Geometry check sheet. Reference: the model listing, model coordinates, mm. A direction names the side the tool comes from. Round coordinates to 2 decimals unless told otherwise and drop trailing zeros. Order: outer loops, then holes, each group sorted by start corner. A loop starts at its lowest first (then second) coordinate and runs counter-clockwise, first axis right, second up. Notation, with made-up numbers: (10, 7.5) - (66, 7.5) arc R27 ccw to (66, 25.5) - close; hole circle Ø7 at (32.5, 49.5). An arc over 180 degrees is marked (long way). Write each question's results on one line, items separated by ' | '.
```python
from build123d import *

# Parameters (mm, degrees)
ESBO_O1_R                = 6.25
RESSALTO_EXTRUS_O1_DEPTH = 16.9
ESBO_O2_R                = 12
RESSALTO_EXTRUS_O2_DEPTH = 1.3
ESBO_O3_R                = 1.6
CORTE_EXTRUS_O1_DEPTH    = 25.884533349
ESBO_O4_R                = 2.45
RESSALTO_EXTRUS_O3_DEPTH = 4.1
ESBO_O5_R                = 0.6
CORTE_EXTRUS_O2_DEPTH    = 1
ESBO_O7_R                = 0.6
CORTE_EXTRUS_O3_DEPTH    = 1


with BuildPart() as part:
    # Esboço1 → Ressalto-extrusão1 (new body)
    with BuildSketch(Plane(origin=(0, 0, 0), x_dir=(1, 0, 0), z_dir=(0, 1, 0))):
        with Locations(Location((0, 0, 0), (0, 0, 270))):
            Circle(ESBO_O1_R)
    extrude(amount=RESSALTO_EXTRUS_O1_DEPTH)

    # Esboço2 → Ressalto-extrusão2 (add)
    with BuildSketch(Plane(origin=(0, 16.9, 0), x_dir=(1, 0, 0), z_dir=(0, 1, 0))):
        with Locations(Location((0, 0, 0), (0, 0, 270))):
            Circle(ESBO_O2_R)
    extrude(amount=RESSALTO_EXTRUS_O2_DEPTH)

    # Esboço3 → Corte-extrusão1 (cut, through all)
    with BuildSketch(Plane(origin=(0, 18.2, 0), x_dir=(1, 0, 0), z_dir=(0, 1, 0))):
        with Locations(Location((0, 9, 0), (0, 0, 270))):
            Circle(ESBO_O3_R)
        with Locations(Location((7.794228634, -4.5, 0), (0, 0, 270))):
            Circle(ESBO_O3_R)
        with Locations(Location((-7.794228634, -4.5, 0), (0, 0, 270))):
            Circle(ESBO_O3_R)
    extrude(amount=-CORTE_EXTRUS_O1_DEPTH, mode=Mode.SUBTRACT)

    # Esboço4 → Ressalto-extrusão3 (add)
    with BuildSketch(Plane(origin=(0, 18.2, 0), x_dir=(1, 0, 0), z_dir=(0, 1, 0))):
        with Locations(Location((0, 0, 0), (0, 0, 270))):
            Circle(ESBO_O4_R)
    extrude(amount=RESSALTO_EXTRUS_O3_DEPTH)

    # Esboço5 → Corte-extrusão2 (cut)
    with BuildSketch(Plane(origin=(0, 22.3, 0), x_dir=(1, 0, 0), z_dir=(0, 1, 0))):
        with Locations(Location((0, 1.4, 0), (0, 0, 270))):
            Circle(ESBO_O5_R)
        with Locations(Location((1.212435565, 0.7, 0), (0, 0, 270))):
            Circle(ESBO_O5_R)
        with Locations(Location((1.212435565, -0.7, 0), (0, 0, 270))):
            Circle(ESBO_O5_R)
        with Locations(Location((0, -1.4, 0), (0, 0, 270))):
            Circle(ESBO_O5_R)
        with Locations(Location((-1.212435565, -0.7, 0), (0, 0, 270))):
            Circle(ESBO_O5_R)
        with Locations(Location((-1.212435565, 0.7, 0), (0, 0, 270))):
            Circle(ESBO_O5_R)
    extrude(amount=-CORTE_EXTRUS_O2_DEPTH, mode=Mode.SUBTRACT)

    # Esboço7 → Corte-extrusão3 (cut)
    with BuildSketch(Plane.XZ):
        with Locations(Location((0, 4.5, 0), (0, 0, 270))):
            Circle(ESBO_O7_R)
        with Locations(Location((1.901782178, 4.078385042, 0), (0, 0, 270))):
            Circle(ESBO_O7_R)
        with Locations(Location((-1.901782178, 4.078385042, 0), (0, 0, 90))):
            Circle(ESBO_O7_R)
        with Locations(Location((-1.901782178, -4.078385042, 0), (0, 0, 270))):
            Circle(ESBO_O7_R)
        with Locations(Location((1.901782178, -4.078385042, 0), (0, 0, 90))):
            Circle(ESBO_O7_R)
        with Locations(Location((0, -4.5, 0), (0, 0, 90))):
            Circle(ESBO_O7_R)
    extrude(amount=-CORTE_EXTRUS_O3_DEPTH, mode=Mode.SUBTRACT)


solid = part.part
```
(1) Material ranges on line 1 (X direction, y = 17.25, z = 4.5); line 2 (X direction, y = 0.45, z = 4.5); line 3 (X direction, y = 21.7, z = -0.7), recorded low to high.
Answers follow:
line 1: -11.12 to -9.39, -6.19 to 6.19, 9.39 to 11.12 | line 2: -4.34 to -2.33, -1.47 to -0.6, 0.6 to 1.47, 2.33 to 4.34 | line 3: -2.35 to -1.81, -0.61 to 0.61, 1.81 to 2.35
(2) Draft check along X on faces 1 (the face through (0, 0, 0)), 2 (the face through (0, 0.5, -5.1)), 3 (the face through (0.736, 20.221, 2.337)). Enter one of: released by +X, released by -X, zero draft, split by the parting line, or undercut.
Answers follow:
face 1: zero draft | face 2: undercut | face 3: split by the parting line
(3) Depth check by flat-ended pin: pin 1 Ø8 at (y, z) = (18, 5) entering from -X; pin 2 Ø0.6 at (x, z) = (0, -1.5) entering from +Y; pin 3 Ø0.6 at (x, z) = (0, -4.5) entering from -Y. Enter the tip coordinate at first touch or a pass-through.
Answers follow:
pin 1: x = -11.96 | pin 2: y = 21.3 | pin 3: y = 1
(4) Section check D-D (x = 8.25). Record the cut outline in (y, z), then the cut area to 3 significant figures.
Answers follow:
outline: (16.9, -8.71) - (18.2, -8.71) - (18.2, 2.97) - (16.9, 2.97) - close; (16.9, 6.03) - (18.2, 6.03) - (18.2, 8.71) - (16.9, 8.71) - close | area: 18.7 mm²
(5) Section check C-C (y = 15.5). Record the cut outline in (x, z).
Answers follow:
outline: circle Ø12.5 at (0, 0)
(6) Section check B-B (z = -10.25). Record the cut outline in (x, y), then the cut area to 3 significant figures.
Answers follow:
outline: (-6.24, 16.9) - (-1, 16.9) - (-1, 18.2) - (-6.24, 18.2) - close; (1, 16.9) - (6.24, 16.9) - (6.24, 18.2) - (1, 18.2) - close | area: 13.6 mm²
(7) Access from +Z, -Z, +X, -X, +Y, -Y to the whole of each face (thin tool, end or side, straight path). Record for faces 4 (the face through (3.604, 17.541, 11.446)), 5 (the face through (-1.03, 21.81, -0.13)), 6 (the face through (-2.08, 0.49, 4.65)).
Answers follow:
face 4: +Y, -Y | face 5: +Y | face 6: -Y
